Could you check a few things on this model? Use its own coordinates, in mm. A direction names the side the tool comes from. Give positions to 0.01 mm unless a question says otherwise; leave off trailing zeros. Order: outer loops, then holes, each group sorted by start corner. A loop starts at its lowest first (then second) coordinate and runs counter-clockwise, first axis right, second up.
from build123d import *

# Parameters (mm, degrees)
SKETCH1_R               = 33
BOSS_EXTRUDE1_DEPTH     = 36
SKETCH2_R               = 30.5
SKETCH2_R_2             = 8
SKETCH2_R_3             = 3
CUT_EXTRUDE2_DEPTH      = 16
SKETCH6_R               = 7.25
SKETCH5_R               = 8
SKETCH7_R               = 30.5
CUT_EXTRUDE3_DEPTH      = 18
SKETCH8_R               = 3
CUT_EXTRUDE4_DEPTH      = 77
SKETCH9_R               = 42.905856896
SKETCH9_R_2             = 32.25
CUT_EXTRUDE5_DEPTH      = 17
CUT_EXTRUDE5_DEPTH_BACK = 17
SKETCH10_R              = 2
CUT_EXTRUDE6_DEPTH      = 17


with BuildPart() as part:
    # Sketch1 → Boss-Extrude1 (new body)
    with BuildSketch(Plane(origin=(0, 0, 0), x_dir=(0, 0, -1), z_dir=(1, 0, 0))):
        Circle(SKETCH1_R)
    extrude(amount=BOSS_EXTRUDE1_DEPTH)

    # Sketch2 → Cut-Extrude2 (cut)
    with BuildSketch(Plane(origin=(36, 0, 0), x_dir=(0, 0, -1), z_dir=(1, 0, 0))):
        Circle(SKETCH2_R)
        Circle(SKETCH2_R_2, mode=Mode.SUBTRACT)
        Circle(SKETCH2_R_2)
        Circle(SKETCH2_R_3, mode=Mode.SUBTRACT)
        Circle(SKETCH2_R_3)
    extrude(amount=-CUT_EXTRUDE2_DEPTH, mode=Mode.SUBTRACT)

    # Sketch6 → Loft2 section 0
    with BuildSketch(Plane(origin=(41, 0, 0), x_dir=(0, 0, -1), z_dir=(1, 0, 0))):
        Circle(SKETCH6_R)
    # Sketch5 → Loft2 section 1
    with BuildSketch(Plane(origin=(20, 0, 0), x_dir=(0, 0, -1), z_dir=(1, 0, 0))):
        Circle(SKETCH5_R)
    loft()

    # Sketch7 → Cut-Extrude3 (cut)
    with BuildSketch(Plane.ZY):
        with Locations(Location((0, 0, 0), (0, 0, 180))):
            Circle(SKETCH7_R)
    extrude(amount=-CUT_EXTRUDE3_DEPTH, mode=Mode.SUBTRACT)

    # Sketch8 → Cut-Extrude4 (cut)
    with BuildSketch(Plane(origin=(41, 0, 0), x_dir=(0, 0, -1), z_dir=(1, 0, 0))):
        Circle(SKETCH8_R)
    extrude(amount=-CUT_EXTRUDE4_DEPTH, mode=Mode.SUBTRACT)

    # Sketch9 → Cut-Extrude5 (cut, two sides)
    with BuildSketch(Plane(origin=(18, 0, 0), x_dir=(0, 0, -1), z_dir=(1, 0, 0))) as cut_extrude5_sk:
        Circle(SKETCH9_R)
        Circle(SKETCH9_R_2, mode=Mode.SUBTRACT)
    extrude(amount=CUT_EXTRUDE5_DEPTH, mode=Mode.SUBTRACT)
    extrude(cut_extrude5_sk.sketch, amount=-CUT_EXTRUDE5_DEPTH_BACK, mode=Mode.SUBTRACT)

    # Sketch10 → Cut-Extrude6 (cut)
    with BuildSketch(Plane(origin=(0, 0, 0), x_dir=(1, 0, 0), z_dir=(0, 1, 0))):
        with Locations(Location((36.300187477, 0, 0), (0, 0, 270))):
            Circle(SKETCH10_R)
    extrude(amount=-CUT_EXTRUDE6_DEPTH, mode=Mode.SUBTRACT)


solid = part.part
Item 1: Imagine slicing it at A-A on z = 0. Give the number of separate pieces and of enclosed holes in the cut face, then the cut area to 3 significant figures.
Findings:
separate pieces: 3
enclosed holes: 0
area: 416 mm2
Item 2: Imagine slicing it at C-C on x = 29. List the corners of the cut face in (y, z) for me.
Findings:
outline: circle Ø64.5 at (0, 0); circle Ø15.36 at (0, 0); hole circle Ø61 at (0, 0); hole circle Ø6 at (0, 0)
Item 3: For faces 1 (the flat face through (20, -6, -6)), 2 (the cylindrical face through (18.24, 9.69, -30.76)), 3 (the flat face through (18, 6, 0)), which set-ups out of +Z, -Z, +X, -X, +Y, -Y let a thin tool reach every point of the face, with its end or its side?
Findings:
face 1: +X
face 2: none
face 3: -X
Item 4: We'd pull the mould along X, two halves only. Please class faces 4 (the cylindrical face through (35.534, -4.826, 1.847)), 5 (the flat face through (41, -2, -3)), 6 (the cylindrical face through (8.874, 29.775, 6.612)), 7 (the flat face through (0, -10, -29)): +X half, -X half, draft (parallel to the pull), parting line (faces both ways), or undercut.
Findings:
face 4: undercut
face 5: +X half
face 6: draft
face 7: -X half
Item 5: Please list where these lines run through material, in increasing order: line 1 along X through (y, z) = (-4, 0); line 2 along Y through (x, z) = (9, 0); line 3 along Y through (x, z) = (25.75, 0).
Findings:
line 1: x = 18 to 34.3, 38.3 to 41
line 2: y = -32.25 to -30.5, 30.5 to 32.25
line 3: y = -32.25 to -30.5, -7.79 to -3, 3 to 7.79, 30.5 to 32.25
Item 6: For pin 1 (4.5 mm diameter, centred on x = 36.3, z = 0, fed in from -Y); pin 2 (3 mm diameter, centred on x = 17.5, z = 19, fed in from -Y); pin 3 (9.5 mm diameter, centred on y = 0, z = 0, fed in from -X), each with a flat end and sliding along its axis, tell me the tip position at first contact or that it passes through.
Findings:
pin 1: stops at y = -33
pin 2: stops at y = -27.09
pin 3: stops at x = 18
Item 7: Imagine slicing it at D-D on z = 9.5. List the corners of the cut face in (x, y) for me.
Findings:
outline: (0, -31.6) - (1, -31.6) - (1, -30.82) - (35, -30.82) - (35, -31.6) - (36, -31.6) - (36, -28.98) - (20, -28.98) - (20, 28.98) - (36, 28.98) - (36, 31.6) - (35, 31.6) - (35, 30.82) - (1, 30.82) - (1, 31.6) - (0, 31.6) - (0, 28.98) - (18, 28.98) - (18, -28.98) - (0, -28.98) - close
Item 8: Imagine slicing it at B-B on y = 20.5. List the corners of the cut face in (x, z) for me, then the cut area to 3 significant figures.
Findings:
outline: (0, -25.86) - (1, -25.86) - (1, -24.9) - (35, -24.9) - (35, -25.86) - (36, -25.86) - (36, -22.58) - (20, -22.58) - (20, 22.58) - (36, 22.58) - (36, 25.86) - (35, 25.86) - (35, 24.9) - (1, 24.9) - (1, 25.86) - (0, 25.86) - (0, 22.58) - (18, 22.58) - (18, -22.58) - (0, -22.58) - close
area: 261 mm2
